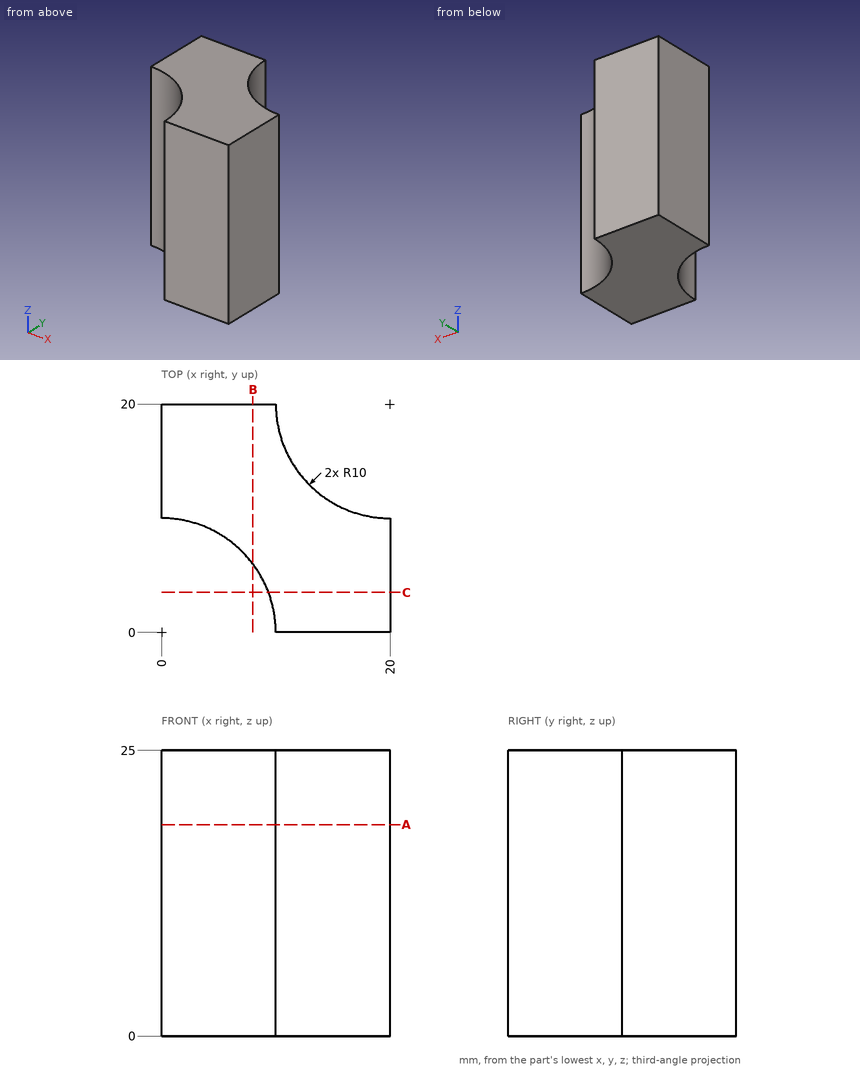
Print and shaded views of the part. All mm, measured from the part's lowest x, y and z. Give positions to 0.01 mm unless a question says otherwise; leave off trailing zeros. Write each loop counter-clockwise with the first axis right and the second up, starting at its lowest first coordinate (ties: lowest second). Pieces come first, ordered by that corner, then holes. Notation, with made-up numbers: M 16,39 L 47,39 A24 cw 47,60 Z; hole C -29,54.25 d2. An arc over 180 degrees is marked long. Use a Markdown table: item, result.
1) Pin check, flat tips, straight feed: pin 1 (1.5 mm diameter, centred on x = 15, z = 4, fed in from +Y); pin 2 (1 mm diameter, centred on y = 13, z = 21, fed in from +X). Stop position of each tip, or through.
Responses:
| item | result |
|---|---|
| pin 1 | stops at y = 11.82 |
| pin 2 | stops at x = 13.39 |
2) Drill centre lines: line 1 (Y direction, x = 5.25, z = 22.5); line 2 (Y direction, x = 14.25, z = 21); line 3 (X direction, y = 12.75, z = 7.25). Where is each one in solid material? Low to high. Write a range as from..to.
Responses:
| item | result |
|---|---|
| line 1 | y = 8.51..20 |
| line 2 | y = 0..11.82 |
| line 3 | x = 0..13.11 |
3) Cut at C-C (y = 3.5). List the corners of the cut face in (x, z).
Responses:
| item | result |
|---|---|
| outline | M 9.37,0 L 20,0 L 20,25 L 9.37,25 Z |
4) Cut at A-A (z = 18.5). List the corners of the cut face in (x, y), and give its area (3 significant figures).
Responses:
| item | result |
|---|---|
| outline | M 0,10 A10 cw 10,0 L 20,0 L 20,10 A10 cw 10,20 L 0,20 Z |
| area | 243 mm2 |
5) Cut at B-B (x = 8). List the corners of the cut face in (y, z), and give its area (3 significant figures).
Responses:
| item | result |
|---|---|
| outline | M 6,0 L 20,0 L 20,25 L 6,25 Z |
| area | 350 mm2 |
